```python
from build123d import *

# Parameters (mm, degrees)
ESBO_O1_W                = 30
ESBO_O1_H                = 30
RESSALTO_EXTRUS_O1_DEPTH = 22.775
CORTE_EXTRUS_O1_DEPTH    = 41.542577927
ESBO_O3_OUTSIDE_W        = 48.998
ESBO_O3_OUTSIDE_H        = 41.63
ESBO_O3_OUTSIDE_W_2      = 30
ESBO_O3_OUTSIDE_H_2      = 30
CORTE_EXTRUS_O2_DEPTH    = 30.010251575
RESSALTO_EXTRUS_O2_DEPTH = 30
ESBO_O5_R                = 3.95
CORTE_EXTRUS_O3_DEPTH    = 32.012511133
CORTE_EXTRUS_O5_START    = -8
ESBO_O8_R                = 6
CORTE_EXTRUS_O5_DEPTH    = 25
RESSALTO_EXTRUS_O6_DEPTH = 30
CORTE_EXTRUS_O11_START   = -21.614745962
CORTE_EXTRUS_O11_DEPTH   = 21.614745962
ESBO_O19_R               = 6.35
CORTE_EXTRUS_O12_DEPTH   = 3.5
ESBO_O20_R               = 3
CORTE_EXTRUS_O13_DEPTH   = 26


with BuildPart() as part:
    # Esboço1 → Ressalto-extrusão1 (new body)
    with BuildSketch(Plane(origin=(0, 0, 0), x_dir=(1, 0, 0), z_dir=(0, 1, 0))):
        Rectangle(ESBO_O1_W, ESBO_O1_H)
    extrude(amount=RESSALTO_EXTRUS_O1_DEPTH)

    # Esboço2 → Corte-extrusão1 (cut, through all)
    with BuildSketch(Plane.XY.offset(15)):
        Polygon((-15, 0), (15, 17.320508076), (15, 0), align=None)
    extrude(amount=-CORTE_EXTRUS_O1_DEPTH, mode=Mode.SUBTRACT)

    # Esboço3 outside → Corte-extrusão2 (cut, through all)
    with BuildSketch(Plane(origin=(-3.75, 6.495190528, 0), x_dir=(0.8660254037844378, 0.5000000000000017, 0), z_dir=(0.5000000000000016, -0.8660254037844377, 0))):
        with Locations((5.694, 0)):
            Rectangle(ESBO_O3_OUTSIDE_W, ESBO_O3_OUTSIDE_H)
        with Locations((4.330127019, 0)):
            Rectangle(ESBO_O3_OUTSIDE_W_2, ESBO_O3_OUTSIDE_H_2, mode=Mode.SUBTRACT)
    extrude(amount=-CORTE_EXTRUS_O2_DEPTH, mode=Mode.SUBTRACT)

    # Esboço4 → Ressalto-extrusão2 (add)
    with BuildSketch(Plane.XY.offset(15)):
        Polygon((-25.469660456, 22.775), (-15, 4.641016151), (-15, 22.775), align=None)
    extrude(amount=-RESSALTO_EXTRUS_O2_DEPTH)

    # Esboço5 → Corte-extrusão3 (cut, through all)
    with BuildSketch(Plane(origin=(-3.75, 6.495190528, 0), x_dir=(-0.8660254037844379, -0.5000000000000013, 0), z_dir=(0.5000000000000013, -0.8660254037844379, 0))):
        with Locations(Location((-4.330131096, -4.077e-06, 0), (0, 0, 180))):
            Circle(ESBO_O5_R)
    extrude(amount=-CORTE_EXTRUS_O3_DEPTH, mode=Mode.SUBTRACT)

    # Esboço8 → Corte-extrusão5 (cut)
    with BuildSketch(Plane(origin=(-3.75, 6.495190528, 0), x_dir=(0.8660254037844379, 0.5000000000000013, 0), z_dir=(0.5000000000000013, -0.8660254037844379, 0)).offset(CORTE_EXTRUS_O5_START)):
        with Locations((4.330131096, 4.077e-06)):
            Circle(ESBO_O8_R)
    extrude(amount=-CORTE_EXTRUS_O5_DEPTH, mode=Mode.SUBTRACT)

    # Esboço16 → Ressalto-extrusão6 (add)
    with BuildSketch(Plane.XY.offset(15)):
        Polygon((9.171355695, 22.775), (30.157076086, 22.775), (30.157076086, 15.275), (11.457076086, 15.275), align=None)
    extrude(amount=-RESSALTO_EXTRUS_O6_DEPTH)

    # Corte-extrusão11: read off the stored shape, not the designer's step
    # Corte-extrusão11 outline → Corte-extrusão11 (cut)
    with BuildSketch(Plane(origin=(0, 22.775, 0), x_dir=(1, 0, 0), z_dir=(0, 1, 0)).offset(CORTE_EXTRUS_O11_START)):
        with BuildLine():
            ThreePointArc((-24.474983506, -14.999998017), (-15.795064462, 6.105795279), (5.221968287, 14.998479898))
            Line((5.221968287, 14.998479898), (5.221968287, 15))
            Line((5.221968287, 15), (-26, 15))
            Line((-26, 15), (-26, -16))
            Line((-26, -16), (-24.47498322, -16))
            Line((-24.47498322, -16), (-24.474983506, -14.999998017))
        make_face()
    extrude(amount=CORTE_EXTRUS_O11_DEPTH, mode=Mode.SUBTRACT)

    # Esboço19 → Corte-extrusão12 (cut)
    with BuildSketch(Plane.XZ.offset(-15.275)):
        with Locations((20.807076086, 0)):
            Circle(ESBO_O19_R)
    extrude(amount=-CORTE_EXTRUS_O12_DEPTH, mode=Mode.SUBTRACT)

    # Esboço20 → Corte-extrusão13 (cut)
    with BuildSketch(Plane.XZ.offset(-18.775)):
        with Locations((20.807076086, 0)):
            Circle(ESBO_O20_R)
    extrude(amount=-CORTE_EXTRUS_O13_DEPTH, mode=Mode.SUBTRACT)


solid = part.part
```
Verification items for the finished model (mm, model axes). A direction names the side the tool comes from. Round coordinates to 2 decimals unless told otherwise and drop trailing zeros. Order: outer loops, then holes, each group sorted by start corner. A loop starts at its lowest first (then second) coordinate and runs counter-clockwise, first axis right, second up. Notation, with made-up numbers: (56.5, -36.75) - (108.5, -36.75) arc R15 cw to (108.5, -13.75) - close; hole circle Ø10 at (79, -19.5). An arc over 180 degrees is marked (long way). Use CSV: the item, a comma, the result in double quotes.
(1) Mould release check, pull along X, two halves, no side actions. Record for faces 5 (the face through (18, 19, -15)), 6 (the face through (15.768, 17, -3.864)), 7 (the face through (-3.654, 6.551, 0.21)): released by +X, released by -X, zero draft, split by the parting line, or undercut.
Entries:
face 5,"zero draft"
face 6,"undercut"
face 7,"released by +X"
(2) Thickness scan on probe 1 along X at (y, z) = (21.75, -1); probe 2 along Z at (x, y) = (-9, 15); probe 3 along Y at (x, z) = (16, -10.25) (3 decimals). Record the ranges inside material, lowest first. Write a range as from..to.
Entries:
probe 1,"-19.85..-14.39, -0.73..17.98, 23.64..30.16"
probe 2,"-11.25..-3.82, 3.82..15"
probe 3,"15.275..22.775"
(3) Gauge pin test, flat ends, axial feed: pin 1 Ø3 at (y, z) = (9.5, -10.5) entering from +X; pin 2 Ø2 at (x, y) = (-8.5, 5) entering from -Z (3 decimals); pin 3 Ø8 at (y, z) = (3.5, 9.5) entering from -X. Record the tip position at first contact, or that the pin passes through.
Entries:
pin 1,"x = 4.05"
pin 2,"z = -12.025"
pin 3,"x = -16.65"
(4) Section check A-A on z = 13.25. Record the boundary of the cut face in (x, y) (3 decimals), and give its area (3 significant figures).
Entries:
outline,"(-24.424, 20.964) - (-12.99, 1.16) - (11.457, 15.275) - (30.157, 15.275) - (30.157, 22.775) - (-24.424, 22.775) - close"
area,"630 mm^2"
(5) Section check B-B on y = 20.25. State how many separate pieces and enclosed holes the cut face has, and give its area (3 significant figures).
Entries:
separate pieces,"1"
enclosed holes,"2"
area,"1,290 mm^2"
(6) Access from +Z, -Z, +X, -X, +Y, -Y to the whole of each face (thin tool, end or side, straight path). Record for faces 1 (the face through (-0.609, 17.546, -1.249)), 2 (the face through (22, 18.775, -3)), 3 (the face through (21, 15.275, 7)), 4 (the face through (9, 22.775, 0)).
Entries:
face 1,"none"
face 2,"-Y"
face 3,"+Z, -Z, +X, -Y"
face 4,"+Z, -Z, +X, -X, +Y"
(7) Section check D-D on y = 2.5. Record the boundary of the cut face in (x, z), and give its area (3 significant figures).
Entries:
outline,"(-13.76, -7.98) arc R30 ccw to (-10.67, -10.25) - (-10.67, 15) - (-13.76, 15) - close"
area,"74.8 mm^2"
(8) Section check C-C on x = 7. Record the boundary of the cut face in (y, z) (3 decimals).
Entries:
outline,"(12.702, -15) - (22.775, -15) - (22.775, 15) - (12.702, 15) - close"
